For this review, take the finished solid that the model builds, in its own axes (mm). Face numbers are marked on the shaded views. Round coordinates to 2 decimals unless told otherwise and drop trailing zeros. Write each loop counter-clockwise with the first axis right and the second up, starting at its lowest first coordinate (ties: lowest second). Pieces come first, ordered by that corner, then holes. Notation, with made-up numbers: (6.5, 15.25) -> (11.5, 15.25) arc R26 cw to (11.5, 47.25) -> close; hole circle Ø2 at (89, 67.25). An arc over 180 degrees is marked (long way). Write each question's results on one line, items separated by ' | '. Start each with the question number.
Item 1: Clearance check with flat-ended pins moving along their axes: pin 1 (2 mm diameter, centred on x = -0.5, z = -5.5, fed in from -Y); pin 2 (6 mm diameter, centred on y = -104, z = 2, fed in from +X) (3 decimals); pin 3 (1 mm diameter, centred on x = 8.5, z = 1, fed in from -Y); pin 4 (3 mm diameter, centred on x = 11, y = -96, fed in from -Z). State where each tip first meets the part, or that it passes through.
Item 2: The part is to be moulded in two halves that separate along Z. For the marked faces 1 and 2, say which applies: +Z half, -Z half, draft (parallel to the pull), parting line (faces both ways), or undercut.
Item 3: To check wall thickness, follow line 1 along X through (y, z) = (-87.5, 1); line 2 along Z through (x, y) = (14.5, -270.5); line 3 along Z through (x, y) = (18, -42). State the ranges of each line that lie inside material, in increasing order.
Item 4: Add section A-A (y = -44). State the section outline as (x, z) points (3 decimals), plus the area to 3 significant figures.
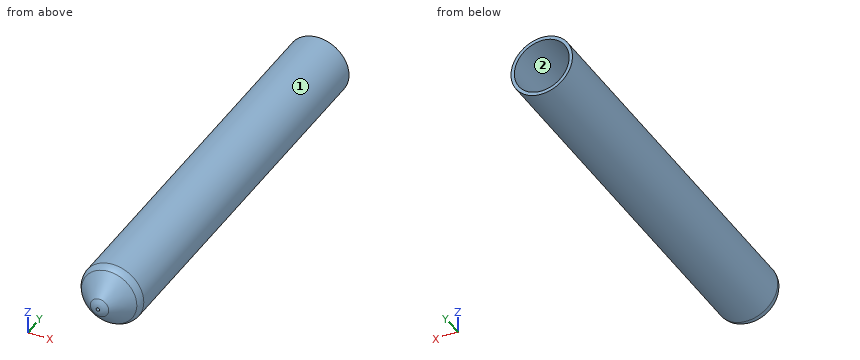
from build123d import *

# Parameters (mm, degrees)
F0_R     = 22.225
F1_DEPTH = 304.8
F2_SIZE  = 17.78
F3_R     = 7.62
F4_R     = 7.62
F6_R     = 19.7961315642
F7_DEPTH = 274.32
F8_R     = 1.2886926547
F9_DEPTH = 304.8


with BuildPart() as f1:
    # F0 (on Front) → F1 (new body)
    with BuildSketch(Plane.XZ):
        Circle(F0_R)
    extrude(amount=F1_DEPTH)

    # F2
    f2_edges = [f1.edges().sort_by_distance(p)[0] for p in [
        (-22.225, -304.8, 0),
    ]]
    chamfer(f2_edges, length=F2_SIZE)

    # F3
    f3_edges = [f1.edges().sort_by_distance(p)[0] for p in [
        (-4.445, -304.8, 0),
    ]]
    fillet(f3_edges, radius=F3_R)

    # F4
    f4_edges = [f1.edges().sort_by_distance(p)[0] for p in [
        (-22.225, -287.02, 0),
    ]]
    fillet(f4_edges, radius=F4_R)

    # F6 (on face) → F7 (cut)
    with BuildSketch(Plane(origin=(0, 0, 0), x_dir=(-1, 0, 0), z_dir=(0, 1, 0))):
        Circle(F6_R)
    extrude(amount=-F7_DEPTH, mode=Mode.SUBTRACT)

    # F8 (on face) → F9 (cut)
    with BuildSketch(Plane.XZ.offset(304.8)):
        Circle(F8_R)
    extrude(amount=-F9_DEPTH, mode=Mode.SUBTRACT)


solid = f1.part
Responses:
1) pin 1: stops at y = -304.08 | pin 2: stops at x = 22.225 | pin 3: stops at y = -301.19 | pin 4: stops at z = -20.09
2) face 1: parting line | face 2: undercut
3) line 1: x = -22.2 to -19.77, 19.77 to 22.2 | line 2: z = -16.84 to -13.48, 13.48 to 16.84 | line 3: z = -13.04 to -8.24, 8.24 to 13.04
4) outline: circle Ø44.45 at (0, 0); hole circle Ø39.592 at (0, 0) | area: 321 mm^2
